Part model, mm, in its own coordinate system. Face numbers are marked on the shaded views. A direction names the side the tool comes from. Give positions to 0.01 mm unless a question says otherwise; leave off trailing zeros. Write each loop counter-clockwise with the first axis right and the second up, starting at its lowest first coordinate (ties: lowest second). Pieces come first, ordered by that corner, then holes. Notation, with made-up numbers: M -26.75,50 L 8.25,50 A25 ccw 8.25,74 Z; hole C -19.75,74 d5. An arc over 180 degrees is marked long. Use CSV: the item, a comma, the result in double quotes. Start each with the question number.
Item 1: Drill centre lines: line 1 (Y direction, x = 0, z = 17.5); line 2 (Y direction, x = 0, z = 14.5); line 3 (Y direction, x = 28.5, z = 22.75). Where is each one in solid material? Low to high. Write a range as [from, to].
Item 2: Which spindle directions (+Z, -Z, +X, -X, +Y, -Y) get a long thin tool onto all of the face, cutting with end or side? Do the marked faces 1, 2 and 3. Say none if no direction does.
Item 3: Cut at A-A (x = 0). List the corners of the cut face in (y, z).
Item 4: Mould opens along Z. For the marked faces 4, 5 and 6 say: released by +Z, released by -Z, zero draft, split by the parting line, or undercut.
Item 5: Pin check, flat tips, straight feed: pin 1 (1.5 mm diameter, centred on x = -24.5, y = 25.5, fed in from -Z); pin 2 (12 mm diameter, centred on x = -33, z = 10.5, fed in from +Y); pin 3 (1 mm diameter, centred on y = 21.5, z = 13, fed in from +X); pin 4 (4 mm diameter, centred on x = 15.5, z = 11, fed in from -Y). Stop position of each tip, or through.
Item 6: Cut at D-D (z = 5.5). List the corners of the cut face in (x, y).
Item 7: Cut at C-C (z = 22.75). List the corners of the cut face in (x, y), then the cut area to 3 significant figures.
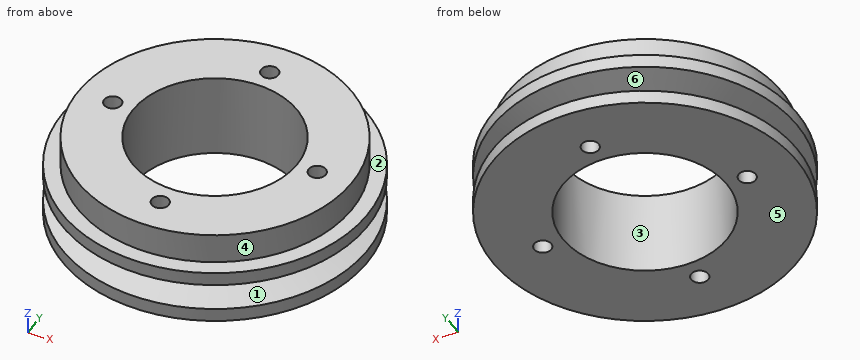
from build123d import *

# Parameters (mm, degrees)
F0_R     = 44.5
F0_R_2   = 40
F0_R_3   = 24
F1_DEPTH = 16
F2_DEPTH = 25
F5_R     = 2.5
F6_DEPTH = 25


with BuildPart() as f1:
    # F0 (on Top) → F1 (new body)
    with BuildSketch(Plane.XY):
        Circle(F0_R)
        Circle(F0_R_2, mode=Mode.SUBTRACT)
        Circle(F0_R_2)
        Circle(F0_R_3, mode=Mode.SUBTRACT)
    extrude(amount=F1_DEPTH)

    # F0 (on Top) → F2 (join)
    with BuildSketch(Plane.XY):
        Circle(F0_R_2)
        Circle(F0_R_3, mode=Mode.SUBTRACT)
    extrude(amount=F2_DEPTH)

    # F3 (on Front) → F4 (revolve, cut)
    with BuildSketch(Plane.XZ):
        Polygon((-34.8, 9.0344123899), (-44.5, 12), (-44.5, 4), (-34.8, 6.9655876101), align=None)
    revolve(axis=Axis((0, 0, -5.6256647222), (0, 0, -1)), mode=Mode.SUBTRACT)

    # F5 (on face) → F6 (cut)
    with BuildSketch(Plane.XY.offset(25)):
        with Locations((0, 30)):
            Circle(F5_R)
        with Locations((30, 0)):
            Circle(F5_R)
        with Locations((0, -30)):
            Circle(F5_R)
        with Locations((-30, 0)):
            Circle(F5_R)
    extrude(amount=-F6_DEPTH, mode=Mode.SUBTRACT)


solid = f1.part
Worked answers:
1,line 1,"y = [-40, -32.5], [-27.5, -24], [24, 27.5], [32.5, 40]"
1,line 2,"y = [-44.5, -32.5], [-27.5, -24], [24, 27.5], [32.5, 44.5]"
1,line 3,"y = [-28.07, -2], [2, 28.07]"
2,face 1,"none"
2,face 2,"+Z"
2,face 3,"+Z, -Z"
3,outline,"M -44.5,0 L -32.5,0 L -32.5,25 L -40,25 L -40,16 L -44.5,16 L -44.5,12 L -34.8,9.03 L -34.8,6.97 L -44.5,4 Z; M -27.5,0 L -24,0 L -24,25 L -27.5,25 Z; M 24,0 L 27.5,0 L 27.5,25 L 24,25 Z; M 32.5,0 L 44.5,0 L 44.5,4 L 34.8,6.97 L 34.8,9.03 L 44.5,12 L 44.5,16 L 40,16 L 40,25 L 32.5,25 Z"
4,face 4,"zero draft"
4,face 5,"released by -Z"
4,face 6,"undercut"
5,pin 1,"stops at z = 0"
5,pin 2,"stops at y = 35.23"
5,pin 3,"stops at x = 39.23"
5,pin 4,"stops at y = -42.32"
6,outline,"C 0,0 d79.19; hole C -30,0 d5; hole C 0,0 d48; hole C 0,-30 d5; hole C 0,30 d5; hole C 30,0 d5"
7,outline,"C 0,0 d80; hole C -30,0 d5; hole C 0,0 d48; hole C 0,-30 d5; hole C 0,30 d5; hole C 30,0 d5"
7,area,"3,140 mm^2"
